Build history of the part. All positions in model axes, mm. A direction names the side the tool comes from. Give positions to 0.01 mm unless a question says otherwise; leave off trailing zeros. Loops run counter-clockwise (first coordinate to the right, second up) from the corner with the lowest first, then second, coordinate; pieces in that order, holes last.
1) Two-plate mould, pull along Y, no slides. Class faces 4 (the cylindrical face through (-11.99, -0.53, -14.38)), 5 (the flat face through (2, 0, -7.4)), 6 (the flat face through (6.2, 7.1, -27.4)): +Y half, -Y half, draft (parallel to the pull), parting line (faces both ways), or undercut.
2) Flat gauge pins, fed straight in: P1, Ø2, axis at x = 0.5, z = -6.5, coming from the -Y side; P2, Ø1.5, axis at y = -5.5, z = -18.5, coming from the +X side; P3, Ø10, axis at y = -9.5, z = -6.5, coming from the +X side. Where does each tip first touch, or does it go through?
3) Band-saw the part on B-B on y = 0. List the corners of the cut face in (x, z), then the cut area to 3 significant figures.
4) Band-saw the part on C-C on z = -22.75. List the corners of the cut face in (x, y).
5) Wall check: line 1 (Y direction, x = 0, z = -22.25); line 2 (Y direction, x = 0, z = -3.5); line 3 (X direction, y = 0, z = -3.25). Give the ranges that are in metal, low to high.
6) Band-saw the part on A-A on x = 0. List the corners of the cut face in (y, z).
7) Band-saw the part on D-D on x = -3.25. List the corners of the cut face in (y, z).
8) 3-axis set-ups, long thin cutter, end or side, ignore diameter. For faces 1 (the flat face through (0, 1.1, -4)), 2 (the flat face through (-7, -10, -1)), 3 (the flat face through (0, 3, 0)): which of +Z, -Z, +X, -X, +Y, -Y reach the whole face in a straight line?
```python
from build123d import *

# Parameters (mm, degrees)
CUT_EXTRUDE_1_DEPTH = 10


with BuildPart() as part:
    # Эскиз1 → Повернуть1 (revolve)
    with BuildSketch(Plane(origin=(0, 0, 0), x_dir=(1, 0, 0), z_dir=(0, 1, 0))):
        Polygon((0, 0), (15, 0), (15, 1), (12, 1), (12, 27.4), (9.25, 27.4), (9.25, 7.4), (0, 7.4), align=None)
    revolve(axis=Axis((0, 0, 0), (0, 0, -1)))

    # Эскиз2 → Вырез-Вытянуть1 (cut)
    # profile 1 of 2: a face of its own
    with BuildSketch(Plane.XY):
        with BuildLine():
            Line((-1.29614814, 1.1), (1.29614814, 1.1))
            ThreePointArc((1.29614814, 1.1), (0, -1.7), (-1.29614814, 1.1))
        make_face()
        with BuildLine():
            ThreePointArc((-1.2, 0.9), (0, -1.5), (1.2, 0.9))
            Line((1.2, 0.9), (-1.2, 0.9))
        make_face(mode=Mode.SUBTRACT)
    # profile 2 of 2: a face of its own
    with BuildSketch(Plane.XY):
        with BuildLine():
            Line((-1.2, 0.9), (1.2, 0.9))
            ThreePointArc((1.2, 0.9), (0, -1.5), (-1.2, 0.9))
        make_face()
    extrude(amount=-CUT_EXTRUDE_1_DEPTH, mode=Mode.SUBTRACT)


solid = part.part
```
Findings below:
1. face 4: parting line
1. face 5: undercut
1. face 6: draft
2. P1: stops at y = -12
2. P2: stops at x = 11.02
2. P3: stops at x = 11.12
3. outline: (-15, -1) - (-12, -1) - (-12, -27.4) - (-9.25, -27.4) - (-9.25, -7.4) - (-1.7, -7.4) - (-1.7, 0) - (-15, 0) - close; (1.7, -7.4) - (9.25, -7.4) - (9.25, -27.4) - (12, -27.4) - (12, -1) - (15, -1) - (15, 0) - (1.7, 0) - close
3. area: 268 mm2
4. outline: circle Ø24 at (0, 0); hole circle Ø18.5 at (0, 0)
5. line 1: y = -12 to -9.25, 9.25 to 12
5. line 2: y = -12 to -1.7, 1.1 to 12
5. line 3: x = -12 to -1.7, 1.7 to 12
6. outline: (-15, -1) - (-12, -1) - (-12, -27.4) - (-9.25, -27.4) - (-9.25, -7.4) - (-1.7, -7.4) - (-1.7, 0) - (-15, 0) - close; (1.1, -7.4) - (9.25, -7.4) - (9.25, -27.4) - (12, -27.4) - (12, -1) - (15, -1) - (15, 0) - (1.1, 0) - close
7. outline: (-14.64, -1) - (-11.55, -1) - (-11.55, -27.4) - (-8.66, -27.4) - (-8.66, -7.4) - (8.66, -7.4) - (8.66, -27.4) - (11.55, -27.4) - (11.55, -1) - (14.64, -1) - (14.64, 0) - (-14.64, 0) - close
8. face 1: +Z, -Z
8. face 2: -Z
8. face 3: +Z, +X, -X, +Y, -Y
